Input: part model. Units: mm. Frame: model coordinates. Round coordinates to 2 decimals unless told otherwise and drop trailing zeros. Write each loop counter-clockwise with the first axis right and the second up, starting at its lowest first coordinate (ties: lowest second). Pieces come first, ordered by that corner, then holes. Notation, with made-up numbers: (14.5, 55.25) - (64.5, 55.25) arc R20 ccw to (64.5, 93.25) - close; hole circle Ø6 at (38, -13.5). An arc over 180 degrees is marked (long way). One line per item, written item: value. Start each with the question number.
```python
from build123d import *

# Parameters (mm, degrees)
F0_W     = 14.2
F0_H     = 13
F1_DEPTH = 0.15
F2_W     = 0.15
F2_H     = 7
F3_DEPTH = 5
F4_R     = 0.5
F6_DEPTH = 25


# Not quite as in the source:
# - a feature names something its author has since deleted; it is built from what else it names


with BuildPart() as f1:
    # F0 (on Top) → F1 (new body)
    with BuildSketch(Plane.XY):
        with BuildLine():
            Line((-13.1, 10.5), (-13.1, 13.5))
            Line((-13.1, 13.5), (-22.1, 13.5))
            Line((-22.1, 13.5), (-22.1, 6.5))
            Line((-22.1, 6.5), (-13.1, 6.5))
            Line((-13.1, 6.5), (-13.1, 9.5))
            Line((-13.1, 9.5), (-14.7, 9.5))
            ThreePointArc((-14.7, 9.5), (-14.9828427125, 9.6171572875), (-15.1, 9.9))
            Line((-15.1, 9.9), (-15.1, 10.1))
            ThreePointArc((-15.1, 10.1), (-14.9828427125, 10.3828427125), (-14.7, 10.5))
            Line((-14.7, 10.5), (-13.1, 10.5))
        make_face()
        with BuildLine():
            Line((13.1, 10.5), (13.1, 13.5))
            Line((13.1, 13.5), (-7.1, 13.5))
            Line((-7.1, 13.5), (-13.1, 13.5))
            Line((-13.1, 13.5), (-13.1, 10.5))
            Line((-13.1, 10.5), (-5.5, 10.5))
            ThreePointArc((-5.5, 10.5), (-5.2171572875, 10.3828427125), (-5.1, 10.1))
            Line((-5.1, 10.1), (-5.1, 9.9))
            ThreePointArc((-5.1, 9.9), (-5.2171572875, 9.6171572875), (-5.5, 9.5))
            Line((-5.5, 9.5), (-13.1, 9.5))
            Line((-13.1, 9.5), (-13.1, 6.5))
            Line((-13.1, 6.5), (-13.1, 0))
            Line((-13.1, 0), (-13.1, -6.5))
            Line((-13.1, -6.5), (-13.1, -9.5))
            Line((-13.1, -9.5), (-5.5, -9.5))
            ThreePointArc((-5.5, -9.5), (-5.2171572875, -9.6171572875), (-5.1, -9.9))
            Line((-5.1, -9.9), (-5.1, -10.1))
            ThreePointArc((-5.1, -10.1), (-5.2171572875, -10.3828427125), (-5.5, -10.5))
            Line((-5.5, -10.5), (-13.1, -10.5))
            Line((-13.1, -10.5), (-13.1, -13.5))
            Line((-13.1, -13.5), (-7.1, -13.5))
            Line((-7.1, -13.5), (13.1, -13.5))
            Line((13.1, -13.5), (13.1, -10.5))
            Line((13.1, -10.5), (5.5, -10.5))
            ThreePointArc((5.5, -10.5), (5.2171572875, -10.3828427125), (5.1, -10.1))
            Line((5.1, -10.1), (5.1, -9.9))
            ThreePointArc((5.1, -9.9), (5.2171572875, -9.6171572875), (5.5, -9.5))
            Line((5.5, -9.5), (13.1, -9.5))
            Line((13.1, -9.5), (13.1, 0))
            Line((13.1, 0), (13.1, 9.5))
            Line((13.1, 9.5), (5.5, 9.5))
            ThreePointArc((5.5, 9.5), (5.2171572875, 9.6171572875), (5.1, 9.9))
            Line((5.1, 9.9), (5.1, 10.1))
            ThreePointArc((5.1, 10.1), (5.2171572875, 10.3828427125), (5.5, 10.5))
            Line((5.5, 10.5), (13.1, 10.5))
        make_face()
        Rectangle(F0_W, F0_H, mode=Mode.SUBTRACT)
    extrude(amount=F1_DEPTH)

    # F2 (on face) → F3 (join)
    with BuildSketch(Plane(origin=(0, 0, 0), x_dir=(1, 0, 0), z_dir=(0, 0, -1))):
        with Locations((-22.025, -10)):
            Rectangle(F2_W, F2_H)
    extrude(amount=F3_DEPTH)

    # F4
    f4_edges = [f1.edges().sort_by_distance(p)[0] for p in [
        (-21.95, 10, 0),
        (-22.1, 10, 0.15),
    ]]
    fillet(f4_edges, radius=F4_R)

    # F5 (on face) → F6 (cut)
    with BuildSketch(Plane(origin=(-22.1, 0, 0), x_dir=(0, -1, 0), z_dir=(-1, 0, 0))):
        with BuildLine():
            Line((-9.9, -3.35), (-10, -3.35))
            Line((-10, -3.35), (-10.1, -3.35))
            ThreePointArc((-10.1, -3.35), (-10.3828427125, -3.4671572875), (-10.5, -3.75))
            Line((-10.5, -3.75), (-10.5, -5))
            Line((-10.5, -5), (-9.5, -5))
            Line((-9.5, -5), (-9.5, -3.75))
            ThreePointArc((-9.5, -3.75), (-9.6171572875, -3.4671572875), (-9.9, -3.35))
        make_face()
    extrude(amount=-F6_DEPTH, mode=Mode.SUBTRACT)


solid = f1.part
```
Q1. Cut plane D-D, the plane y = 9. Output: boundary loops of the cut face in (x, z), and give its area (3 significant figures).
Q2. Cut plane A-A, the plane x = -4. Output: boundary loops of the cut face in (y, z), and give its area (3 significant figures).
Q3. Contact query for flat-ended pins moving along their axis: pin 1 Ø1.5 at (x, y) = (1, -4) entering from +Z; pin 2 Ø6 at (x, y) = (-13.5, -5.5) entering from +Z. Output: stop coordinate, or through.
Q4. Cut plane C-C, the plane x = 11. Output: boundary loops of the cut face in (y, z), and give its area (3 significant figures).
Q5. Cut plane B-B, the plane z = -4.35. Output: boundary loops of the cut face in (x, y), and give its area (3 significant figures).
Q6. Material intervals for probe 1 along Z at (x, y) = (-7, 7.5), sorted ascending. Write a range as from..to.
A:
1. outline: (-22.1, -5) - (-21.95, -5) - (-21.95, -0.5) arc R0.5 cw to (-21.45, 0) - (13.1, 0) - (13.1, 0.15) - (-21.6, 0.15) arc R0.5 ccw to (-22.1, -0.35) - close
1. area: 6.03 mm²
2. outline: (-13.5, 0) - (-6.5, 0) - (-6.5, 0.15) - (-13.5, 0.15) - close; (6.5, 0) - (13.5, 0) - (13.5, 0.15) - (6.5, 0.15) - close
2. area: 2.10 mm²
3. pin 1: passes through
3. pin 2: stops at z = 0.15
4. outline: (-13.5, 0) - (-10.5, 0) - (-10.5, 0.15) - (-13.5, 0.15) - close; (-9.5, 0) - (9.5, 0) - (9.5, 0.15) - (-9.5, 0.15) - close; (10.5, 0) - (13.5, 0) - (13.5, 0.15) - (10.5, 0.15) - close
4. area: 3.75 mm²
5. outline: (-22.1, 6.5) - (-21.95, 6.5) - (-21.95, 9.5) - (-22.1, 9.5) - close; (-22.1, 10.5) - (-21.95, 10.5) - (-21.95, 13.5) - (-22.1, 13.5) - close
5. area: 0.900 mm²
6. probe 1: z = 0..0.15
